Verification items for the finished model (mm, model axes). A direction names the side the tool comes from. Give positions to 0.01 mm unless a question says otherwise; leave off trailing zeros. Loops run counter-clockwise (first coordinate to the right, second up) from the corner with the lowest first, then second, coordinate; pieces in that order, holes last. Notation, with made-up numbers: (-35.5, 86.5) -> (-1.5, 86.5) arc R14 cw to (-1.5, 111.5) -> close; hole circle Ø6 at (41, 84). An arc over 180 degrees is marked (long way). Answer in a Markdown table with one row per item. Add a question column.
Q1. Material ranges on probe 1 along Y at (x, z) = (31, -53); probe 2 along Z at (x, y) = (35.5, 103); probe 3 along Z at (x, y) = (4, 12.5), recorded low to high.
Q2. Release check for a two-part mould opening along Z. For faces 4 (the face through (25, 69, -140)), 5 (the face through (25, 61, 0)), 6 (the face through (24.65, 127.15, -13.01)) record: pulls with the +Z half, pulls with the -Z half, needs draft (parallel to the pull), parting line crosses it, or undercut.
Q3. Section check A-A on y = 34. Enter the section's corners in (x, z), and give its area (3 significant figures).
Q4. Section check C-C on x = 48. Enter the section's corners in (y, z).
Q5. Set-up check for faces 1 (the face through (25, 0, -69)), 2 (the face through (54.437, 4.324, -2.854)), 3 (the face through (25, 130, -71)): record each of +Z, -Z, +X, -X, +Y, -Y from which the full face is reachable in a straight line by a thin tool's end or side.
Q6. Section check B-B on z = -63. Enter the section's corners in (x, y), and give its area (3 significant figures).
Q7. Section check D-D on y = 5. Enter the section's corners in (x, z), and give its area (3 significant figures).
```python
from build123d import *

# Parameters (mm, degrees)
EXTRUDE_1_DEPTH = 50
SKETCH_2_R      = 2.25
EXTRUDE_2_DEPTH = 9


with BuildPart() as part:
    # 草图1 → 凸台-拉伸1 (new body)
    with BuildSketch(Plane(origin=(0, 0, 0), x_dir=(0, 0, -1), z_dir=(1, 0, 0))):
        with BuildLine():
            Line((0, 0), (140, 0))
            Line((140, 0), (140, 140))
            Line((140, 140), (20, 140))
            ThreePointArc((20, 140), (5.857864376, 134.142135624), (0, 120))
            Line((0, 120), (0, 0))
        make_face()
        with BuildLine():
            Line((20, 10), (120, 10))
            ThreePointArc((120, 10), (127.071067812, 12.928932188), (130, 20))
            Line((130, 20), (130, 120))
            ThreePointArc((130, 120), (127.071067812, 127.071067812), (120, 130))
            Line((120, 130), (20, 130))
            ThreePointArc((20, 130), (12.928932188, 127.071067812), (10, 120))
            Line((10, 120), (10, 20))
            ThreePointArc((10, 20), (12.928932188, 12.928932188), (20, 10))
        make_face(mode=Mode.SUBTRACT)
    extrude(amount=EXTRUDE_1_DEPTH)

    # 草图2 → 凸台-拉伸2 (add)
    with BuildSketch(Plane(origin=(50, 0, 0), x_dir=(0, 0, -1), z_dir=(1, 0, 0))):
        with Locations(Location((5, 5, 0), (0, 0, 180))):
            Circle(SKETCH_2_R)
        with Locations(Location((135, 5, 0), (0, 0, 180))):
            Circle(SKETCH_2_R)
        with Locations(Location((135, 135, 0), (0, 0, 180))):
            Circle(SKETCH_2_R)
    extrude(amount=EXTRUDE_2_DEPTH)


solid = part.part
```
Taken from the geometry:
| question | item | result |
|---|---|---|
| 1 | probe 1 | y = 0 to 10, 130 to 140 |
| 1 | probe 2 | z = -140 to -130, -10 to 0 |
| 1 | probe 3 | z = -140 to -126.61, -13.39 to 0 |
| 2 | face 4 | pulls with the -Z half |
| 2 | face 5 | pulls with the +Z half |
| 2 | face 6 | undercut |
| 3 | outline | (0, -140) -> (50, -140) -> (50, -130) -> (0, -130) -> close; (0, -10) -> (50, -10) -> (50, 0) -> (0, 0) -> close |
| 3 | area | 1,000 mm² |
| 4 | outline | (0, -140) -> (140, -140) -> (140, -20) arc R20 ccw to (120, 0) -> (0, 0) -> close; hole (10, -120) arc R10 ccw to (20, -130) -> (120, -130) arc R10 ccw to (130, -120) -> (130, -20) arc R10 ccw to (120, -10) -> (20, -10) arc R10 ccw to (10, -20) -> close |
| 5 | face 1 | +Z, -Z, +X, -X, -Y |
| 5 | face 2 | +X |
| 5 | face 3 | +X, -X |
| 6 | outline | (0, 0) -> (50, 0) -> (50, 10) -> (0, 10) -> close; (0, 130) -> (50, 130) -> (50, 140) -> (0, 140) -> close |
| 6 | area | 1,000 mm² |
| 7 | outline | (0, -140) -> (50, -140) -> (50, -137.25) -> (59, -137.25) -> (59, -132.75) -> (50, -132.75) -> (50, -7.25) -> (59, -7.25) -> (59, -2.75) -> (50, -2.75) -> (50, 0) -> (0, 0) -> close |
| 7 | area | 7,080 mm² |
